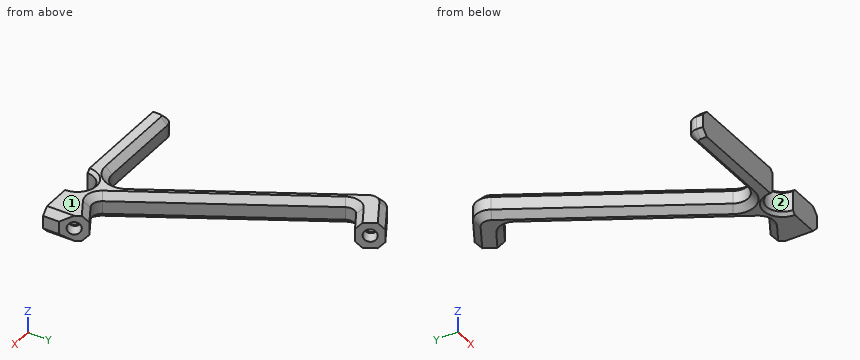
Autodesk Fusion 360 part; units mm, degrees
sketch "Sketch1" plane through (0, 0, 0) normal (0, 0, 1) x (1, 0, 0)
  line L0 (0, 0) -> (55.9904, 0)
  line L1 (55.9904, 0) -> (55.9904, 5)
  line L2 (30.0096, 5) -> (3, 5)
  line L3 (0, 5) -> (0, 0)
  line L4 (34.3397, 12.5) -> (2.5, 67.6481)
  line L5 (41.5566, 0) -> (125.219, 0) construction
  line L6 (9.8301, 64.9519) -> (41.8301, 9.5263)
  line L7 (4.3301, 74.4782) -> (12.9904, 79.4782)
  line L8 (12.9904, 79.4782) -> (16.9904, 72.55)
  line L9 (16.9904, 72.55) -> (10.9282, 69.05)
  line L10 (14.9904, 76.0141) -> (36.6637, 88.5272) construction
  line L11 (0, 2) -> (0, 0) construction
  line L12 (55.9904, 5) -> (51.9904, 11.9282)
  line L13 (51.9904, 11.9282) -> (45.9282, 8.4282)
  arc A0 (4.3301, 74.4782) -> (2.5, 67.6481) centre (6.8301, 70.1481) ccw
  arc A1 (3, 5) -> (0, 2) centre (3, 2) ccw
  arc A2 (30.0096, 5) -> (34.3397, 12.5) centre (30.0096, 10) ccw
  arc A3 (41.8301, 9.5263) -> (45.9282, 8.4282) centre (44.4282, 11.0263) ccw
  arc A4 (10.9282, 69.05) -> (9.8301, 64.9519) centre (12.4282, 66.4519) ccw
  arc A5 (44.1423, 0) -> (34.1423, 0) centre (39.1423, 0) ccw
  line L14 (53.9904, 8.4641) -> (45.1077, 3.3357) construction
  point P0 (0, 71.9782)
  dimension "d1" = 5
  dimension "d2" = 120
  dimension "d3" = 5
  dimension "d4" = 8
  dimension "d8" = 8
  dimension "d9" = 5
  dimension "d10" = 3
  dimension "d11" = 5
  dimension "d12" = 3
  dimension "d13" = 3
  dimension "d24" = 5
  dimension "d30" = 10
  dimension "d31" = 5
  dimension "d32" = 78
extrude "Extrude1" add sketch "Sketch1" along normal blind 8 contours L0 L1 L2 L3 L4 L6 L7 L8 L9 L12 L13 A0 A1 A2 A3 A4 A5
sketch "Sketch2" plane through (44.1578, 25.4945, 0) normal (0.866, 0.5, 0) x (-0.5, 0.866, 0)
  line L0 (54.3349, 0) -> (62.3349, 0)
  line L1 (62.3349, 0) -> (62.3349, 8)
  line L2 (62.3349, 8) -> (54.3349, 8)
  line L3 (54.3349, 8) -> (54.3349, 0)
  line L4 (-23.6651, 0) -> (-15.6651, 0) construction
  line L5 (-15.6651, 0) -> (-15.6651, 8) construction
  line L6 (-15.6651, 8) -> (-23.6651, 8) construction
  line L7 (-23.6651, 8) -> (-23.6651, 0) construction
  line L8 (54.3349, 8) -> (62.3349, 0) construction
  line L9 (62.3349, 8) -> (54.3349, 0) construction
  line L10 (-23.6651, 8) -> (-15.6651, 0) construction
  line L11 (-15.6651, 8) -> (-23.6651, 0) construction
  circle A0 centre (-19.6651, 4) radius 2
  circle A1 centre (58.3349, 4) radius 2
  circle A2 centre (-19.6651, 4) radius 1.6
  circle A3 centre (58.3349, 4) radius 1.6
  dimension "d16" = 4
  dimension "d17" = 4
  dimension "d26" = 3.2
  dimension "d27" = 3.2
extrude "Extrude2" cut sketch "Sketch2" against normal blind 4 contours A0 | A1 | A2 | A3
extrude "Extrude3" cut sketch "Sketch2" against normal blind 10 contours A2 | A3
chamfer "Chamfer1" distance 2 angle 45 26 edges at (16.5048, 5, 8) (34.3397, 7.5, 8) (18.4199, 40.074, 8) (2.0005, 71.4422, 8) (8.6602, 76.9782, 8) (0, 1, 8) (0.8787, 4.1213, 8) (25.8301, 37.2391, 8) (43.6517, 8.1285, 8) (48.9593, 10.1782, 8) (13.9593, 70.8, 8) (9.5304, 67.2284, 8) (25.8301, 37.2391, 0) (9.5304, 67.2284, 0) (13.9593, 70.8, 0) (48.9593, 10.1782, 0) (43.6517, 8.1285, 0) (18.4199, 40.074, 0) (34.3397, 7.5, 0) (16.5048, 5, 0) (0.8787, 4.1213, 0) (0, 1, 0) (8.6602, 76.9782, 0) (2.0005, 71.4422, 0) (55.9904, 2.5, 8) (55.9904, 2.5, 0)
chamfer "Chamfer2" distance 1 angle 45 2 edges at (39.1423, 5, 0) (39.1423, 5, 8)
The listing builds one solid part. Answer for the finished solid, in the listing's coordinates (mm). Face numbers are marked on the shaded views. Round coordinates to 2 decimals unless told otherwise and drop trailing zeros. Order: outer loops, then holes, each group sorted by start corner. A loop starts at its lowest first (then second) coordinate and runs counter-clockwise, first axis right, second up. Notation, with made-up numbers: (69, -30.75) - (118, -30.75) arc R16 cw to (118, -6.75) - close; hole circle Ø9 at (57.25, 27). An arc over 180 degrees is marked (long way). Put each result on its own line as item: value. Start each with the question number.
(1) Find section A-A (x = 29). Give the vertices of the cut face in (y, z).
(2) Find section B-B (y = 27). Give the vertices of the cut face in (x, z), plus the area to 3 significant figures.
(3) Determine the mould class of the marked faces 1 and 2 for opening direction X: released by +X, released by -X, zero draft, split by the parting line, or undercut.
(4) Straight lines are drawn through the part: probe 1 along Y at (x, z) = (15, 4.25); probe 2 along Z at (x, y) = (50, 4.5); probe 3 along Y at (x, z) = (10.5, 2.75). For each, find the intervals that lie inside material, in ascending order. Write a range as from..to.
(5) Given P1, Ø1, axis at y = 51, z = 1.5, coming from the -X side; P2, Ø2, axis at y = 18.5, z = 2.5, coming from the +X side; P3, Ø1.2, axis at x = 22.5, z = 4, coming from the +Y side, each flat-ended and moving along its own axis, determine where each tip first touches the part or whether it passes through.
Reply:
1. outline: (0, 0) - (3, 0) - (5, 2) - (5, 6) - (3, 8) - (0, 8) - close; (21.75, 2) - (25.75, 0) - (27.75, 0) - (31.75, 2) - (31.75, 6) - (27.75, 8) - (25.75, 8) - (21.75, 6) - close
2. outline: (25.97, 2) - (28.28, 0) - (29.43, 0) - (31.74, 2) - (31.74, 6) - (29.43, 8) - (28.28, 8) - (25.97, 6) - close
2. area: 37.0 mm^2
3. face 1: zero draft
3. face 2: undercut
4. probe 1: 0..5, 46..56, 71.4..73.73
4. probe 2: 0..3.3, 4.7..8
4. probe 3: 0..5, 53.79..63.79, 68.75..72.27, 74.57..78.04
5. P1: x = 12.04
5. P2: x = 37.23
5. P3: y = 44.05
